Geometry check sheet. Reference: the model listing, model coordinates, mm. A direction names the side the tool comes from. Round coordinates to 2 decimals unless told otherwise and drop trailing zeros. Order: outer loops, then holes, each group sorted by start corner. A loop starts at its lowest first (then second) coordinate and runs counter-clockwise, first axis right, second up. Notation, with made-up numbers: (56.25, -9) - (97.25, -9) arc R30 cw to (97.25, 27) - close; hole circle Ø1 at (-34.5, -30). An arc over 180 degrees is marked (long way). Write each question's results on one line, items separated by ' | '.
```python
from build123d import *

# Parameters (mm, degrees)
F1_DEPTH  = 23
F5_D      = 6
F6_D      = 6
F7_START  = 14.6
F2_W      = 5.5
F2_H      = 10.4
F7_DEPTH  = 29.6
F9_R      = 8.5
F9_R_2    = 6
F10_DEPTH = 7
F8_R      = 8.5
F8_R_2    = 6
F11_DEPTH = 7
F12_START = -14.6
F12_DEPTH = 30.8


with BuildPart() as f1:
    # F0 (on Top) → F1 (new body)
    with BuildSketch(Plane.XY):
        with BuildLine():
            Line((37.5, 33), (-37.5, 33))
            Line((-37.5, 33), (-37.5, 0))
            Line((-37.5, 0), (-14.1, 0))
            ThreePointArc((-14.1, 0), (0, 14.1), (14.1, 0))
            Line((14.1, 0), (37.5, 0))
            Line((37.5, 0), (37.5, 33))
        make_face()
    extrude(amount=F1_DEPTH)

    # F5 (through all)
    with Locations(Plane.XZ):
        with Locations((-25.8, 11.5)):
            Hole(F5_D / 2)

    # F6 (through all)
    with Locations(Plane.XZ):
        with Locations((25.8, 11.5)):
            Hole(F6_D / 2)

    # F2 (on Right) → F7 (cut)
    with BuildSketch(Plane.YZ.offset(F7_START)):
        with Locations((8.363037575, 11.5)):
            Rectangle(F2_W, F2_H)
        with Locations((22.25, 11.5)):
            Rectangle(F2_W, F2_H)
    extrude(amount=F7_DEPTH, mode=Mode.SUBTRACT)

    # F9 (on face) → F10 (cut)
    with BuildSketch(Plane(origin=(0, 33, 0), x_dir=(-1, 0, 0), z_dir=(0, 1, 0))):
        with Locations((-25.8, 11.5)):
            Circle(F9_R)
        with Locations((-25.8, 11.5)):
            Circle(F9_R_2, mode=Mode.SUBTRACT)
    extrude(amount=-F10_DEPTH, mode=Mode.SUBTRACT)

    # F8 (on face) → F11 (cut)
    with BuildSketch(Plane(origin=(0, 33, 0), x_dir=(-1, 0, 0), z_dir=(0, 1, 0))):
        with Locations((25.8, 11.5)):
            Circle(F8_R)
        with Locations((25.8, 11.5)):
            Circle(F8_R_2, mode=Mode.SUBTRACT)
    extrude(amount=-F11_DEPTH, mode=Mode.SUBTRACT)

    # F2 (on Right) → F12 (cut)
    with BuildSketch(Plane.YZ.offset(F12_START)):
        with Locations((8.363037575, 11.5)):
            Rectangle(F2_W, F2_H)
        with Locations((22.25, 11.5)):
            Rectangle(F2_W, F2_H)
    extrude(amount=-F12_DEPTH, mode=Mode.SUBTRACT)


solid = f1.part
```
(1) Section check B-B (y = 30.5). Record the cut outline in (x, z), then the cut area to 3 significant figures.
Answers follow:
outline: (-37.5, 0) - (37.5, 0) - (37.5, 23) - (-37.5, 23) - close; circle Ø12 at (-25.8, 11.5); circle Ø12 at (25.8, 11.5); hole circle Ø17 at (-25.8, 11.5); hole circle Ø6 at (-25.8, 11.5); hole circle Ø17 at (25.8, 11.5); hole circle Ø6 at (25.8, 11.5) | area: 1,440 mm²
(2) Section check A-A (x = -16.5). Record the cut outline in (y, z), then the cut area to 3 significant figures.
Answers follow:
outline: (0, 0) - (33, 0) - (33, 23) - (0, 23) - close; hole (5.61, 6.3) - (11.11, 6.3) - (11.11, 16.7) - (5.61, 16.7) - close; hole (19.5, 6.3) - (25, 6.3) - (25, 16.7) - (19.5, 16.7) - close | area: 645 mm²
(3) Access from +Z, -Z, +X, -X, +Y, -Y to the whole of each face (thin tool, end or side, straight path). Record for faces 1 (the face through (-14.6, 22, 12)), 2 (the face through (-23.96, 29.55, 3.2)), 3 (the face through (-37.5, 17, 11)), 4 (the face through (28, 25, 14)).
Answers follow:
face 1: -X | face 2: +Y | face 3: +Z, -Z, -X, +Y, -Y | face 4: +X
(4) Material ranges on line 1 (Z direction, x = 25.8, y = 28.25); line 2 (Y direction, x = 17.5, z = 15.25); line 3 (Y direction, x = -31, z = 6.75), recorded low to high.
Answers follow:
line 1: 0 to 3, 5.5 to 8.5, 14.5 to 17.5, 20 to 23 | line 2: 0 to 5.61, 11.11 to 19.5, 25 to 33 | line 3: 0 to 5.61, 11.11 to 19.5, 25 to 26
(5) Draft check along Z on faces 5 (the face through (-1, 17, 0)), 6 (the face through (28, 11.113, 14)), 7 (the face through (28, 0, 9)). Enter one of: released by +Z, released by -Z, zero draft, split by the parting line, or undercut.
Answers follow:
face 5: released by -Z | face 6: undercut | face 7: zero draft
(6) Section check C-C (y = 4). Record the cut outline in (x, z).
Answers follow:
outline: (-37.5, 0) - (-13.52, 0) - (-13.52, 23) - (-37.5, 23) - close; (13.52, 0) - (37.5, 0) - (37.5, 23) - (13.52, 23) - close; hole circle Ø6 at (-25.8, 11.5); hole circle Ø6 at (25.8, 11.5)
(7) Depth check by flat-ended pin: pin 1 Ø5.5 at (x, z) = (25.8, 11.5) entering from +Y; pin 2 Ø6 at (x, z) = (-2, 5) entering from -Y. Enter the tip coordinate at first touch or a pass-through.
Answers follow:
pin 1: through | pin 2: y = 13.18
